Design review of the part built by this model. Coordinates are the model's own, in mm. Coordinates: 2 decimals unless noted, no trailing zeros. Loops run counter-clockwise (first coordinate to the right, second up) from the corner with the lowest first, then second, coordinate; pieces in that order, holes last. Notation, with made-up numbers: (65.5, 15) -> (77.5, 15) arc R16 cw to (77.5, 45) -> close; hole circle Ø6 at (-30.5, 87.5). An arc over 180 degrees is marked (long way). Answer in a Markdown table with one row per item.
```python
from build123d import *

# Parameters (mm, degrees)
SKETCH_2_W          = 6.5
SKETCH_2_H          = 25
EXTRUDE_1_DEPTH     = 73.5
FILLET_1_R          = 1
SKETCH_3_R          = 1.6
CUT_EXTRUDE_1_DEPTH = 75.838158716
CHAMFER_2_SIZE      = 2
SKETCH_4_R          = 4.25
CUT_EXTRUDE_2_DEPTH = 75.838158716


with BuildPart() as part:
    # 草图2 → 凸台-拉伸1 (new, symmetric)
    with BuildSketch(Plane.XY):
        Rectangle(SKETCH_2_W, SKETCH_2_H)
    extrude(amount=EXTRUDE_1_DEPTH, both=True)

    # 圆角1
    fillet_1_edges = [part.edges().sort_by_distance(p)[0] for p in [
        (-3.25, -12.5, 0),
    ]]
    fillet(fillet_1_edges, radius=FILLET_1_R)

    # 草图3 → 切除-拉伸1 (cut, through all)
    with BuildSketch(Plane.ZY.offset(3.25)):
        with Locations(Location((63.5, -2.5, 0), (0, 0, 270))):
            Circle(SKETCH_3_R)
        with Locations(Location((21.166666667, -2.5, 0), (0, 0, 270))):
            Circle(SKETCH_3_R)
        with Locations(Location((-21.166666667, -2.5, 0), (0, 0, 270))):
            Circle(SKETCH_3_R)
        with Locations(Location((-63.5, -2.5, 0), (0, 0, 270))):
            Circle(SKETCH_3_R)
    extrude(amount=-CUT_EXTRUDE_1_DEPTH, mode=Mode.SUBTRACT)

    # 倒角2
    chamfer_2_edges = [part.edges().sort_by_distance(p)[0] for p in [
        (-3.25, -0.9, 63.5),
        (-3.25, -0.9, 21.166666667),
        (-3.25, -0.9, -21.166666667),
        (-3.25, -0.9, -63.5),
    ]]
    chamfer(chamfer_2_edges, length=CHAMFER_2_SIZE)

    # 草图4 → 切除-拉伸2 (cut, through all)
    with BuildSketch(Plane.ZY.offset(3.25)):
        with Locations((-63.5, 12.5)):
            Circle(SKETCH_4_R)
        with Locations((63.5, 12.5)):
            Circle(SKETCH_4_R)
    extrude(amount=-CUT_EXTRUDE_2_DEPTH, mode=Mode.SUBTRACT)


solid = part.part
```
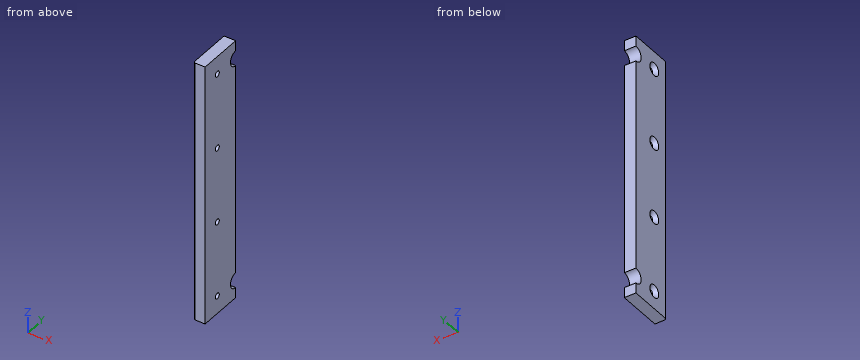
(1) For pin 1 (3.5 mm diameter, centred on y = -2.5, z = 21.17, fed in from +X), flat-tipped, find the tip position at first contact; note if it passes through.
Evaluation:
| item | result |
|---|---|
| pin 1 | stops at x = 3.25 |
(2) To check wall thickness, follow probe 1 along Z at (x, y) = (1.8, -2.5); probe 2 along Z at (x, y) = (2.25, -2.75); probe 3 along Z at (x, y) = (-0.25, 9.25). State the ranges of each line that lie inside material, in increasing order.
Evaluation:
| item | result |
|---|---|
| probe 1 | z = -73.5 to -65.1, -61.9 to -22.77, -19.57 to 19.57, 22.77 to 61.9, 65.1 to 73.5 |
| probe 2 | z = -73.5 to -65.08, -61.92 to -22.75, -19.59 to 19.59, 22.75 to 61.92, 65.08 to 73.5 |
| probe 3 | z = -73.5 to -66.24, -60.76 to 60.76, 66.24 to 73.5 |
(3) Take a section at B-B on y = -2.5. Give the boundary of the cut face in (x, z).
Evaluation:
| item | result |
|---|---|
| outline | (-3.25, -73.5) -> (3.25, -73.5) -> (3.25, -65.1) -> (-1.25, -65.1) -> (-3.25, -67.1) -> close; (-3.25, -59.9) -> (-1.25, -61.9) -> (3.25, -61.9) -> (3.25, -22.77) -> (-1.25, -22.77) -> (-3.25, -24.77) -> close; (-3.25, -17.57) -> (-1.25, -19.57) -> (3.25, -19.57) -> (3.25, 19.57) -> (-1.25, 19.57) -> (-3.25, 17.57) -> close; (-3.25, 24.77) -> (-1.25, 22.77) -> (3.25, 22.77) -> (3.25, 61.9) -> (-1.25, 61.9) -> (-3.25, 59.9) -> close; (-3.25, 67.1) -> (-1.25, 65.1) -> (3.25, 65.1) -> (3.25, 73.5) -> (-3.25, 73.5) -> close |
(4) Take a section at A-A on z = -63.5. Give the boundary of the cut face in (x, y).
Evaluation:
| item | result |
|---|---|
| outline | (-3.25, -11.5) arc R1 ccw to (-2.25, -12.5) -> (3.25, -12.5) -> (3.25, -4.1) -> (-1.25, -4.1) -> (-3.25, -6.1) -> close; (-3.25, 1.1) -> (-1.25, -0.9) -> (3.25, -0.9) -> (3.25, 8.25) -> (-3.25, 8.25) -> close |
(5) Take a section at C-C on x = 0. Give the boundary of the cut face in (y, z).
Evaluation:
| item | result |
|---|---|
| outline | (-12.5, -73.5) -> (12.5, -73.5) -> (12.5, -67.75) arc R4.25 cw to (12.5, -59.25) -> (12.5, 59.25) arc R4.25 cw to (12.5, 67.75) -> (12.5, 73.5) -> (-12.5, 73.5) -> close; hole circle Ø3.2 at (-2.5, -63.5); hole circle Ø3.2 at (-2.5, -21.17); hole circle Ø3.2 at (-2.5, 21.17); hole circle Ø3.2 at (-2.5, 63.5) |
